```python
from build123d import *

# Parameters (mm, degrees)
BOSS_EXTRUDE1_DEPTH     = 20
BOSS_EXTRUDE4_START     = -30
BOSS_EXTRUDE4_DEPTH     = 42
SKETCH10_W              = 40
SKETCH10_H              = 22
CUT_EXTRUDE3_DEPTH      = 147
SKETCH11_R              = 15
BOSS_EXTRUDE5_DEPTH     = 18
CUT_EXTRUDE4_REACH      = 177
SKETCH12_R              = 10
FILLET1_R               = 3
SKETCH13_R              = 4
CUT_EXTRUDE5_DEPTH      = 86
CUT_EXTRUDE5_DEPTH_BACK = 86
CUT_EXTRUDE7_REACH      = 177
SKETCH16_R              = 6.5


with BuildPart() as part:
    # Sketch1 → Boss-Extrude1 (new body)
    with BuildSketch(Plane(origin=(0, 0, 0), x_dir=(1, 0, 0), z_dir=(0, 1, 0))):
        with BuildLine():
            Line((-80, 30), (80, 30))
            ThreePointArc((80, 30), (83.535533906, 28.535533906), (85, 25))
            Line((85, 25), (85, -25))
            ThreePointArc((85, -25), (83.535533906, -28.535533906), (80, -30))
            Line((80, -30), (-80, -30))
            ThreePointArc((-80, -30), (-83.535533906, -28.535533906), (-85, -25))
            Line((-85, -25), (-85, 25))
            ThreePointArc((-85, 25), (-83.535533906, 28.535533906), (-80, 30))
        make_face()
    extrude(amount=BOSS_EXTRUDE1_DEPTH)

    # Sketch2 → Boss-Extrude4 (add)
    with BuildSketch(Plane.XY.offset(BOSS_EXTRUDE4_START)):
        with BuildLine():
            Line((-17.90827935, 157), (42.09172065, 157))
            Line((42.09172065, 157), (42.09172065, 85))
            Line((42.09172065, 85), (-7.90827935, 85))
            Line((-7.90827935, 85), (-7.90827935, 45))
            Line((-7.90827935, 45), (15, 20))
            Line((15, 20), (37.90827935, 45))
            Line((37.90827935, 45), (42.09172065, 45))
            Line((42.09172065, 45), (42.09172065, 25))
            ThreePointArc((42.09172065, 25), (43.556186744, 21.464466094), (47.09172065, 20))
            Line((47.09172065, 20), (50, 20))
            Line((50, 20), (50, 17))
            Line((50, 17), (-58, 17))
            Line((-58, 17), (-58, 20))
            Line((-58, 20), (-57.90827935, 20))
            ThreePointArc((-57.90827935, 20), (-54.372745445, 21.464466094), (-52.90827935, 25))
            Line((-52.90827935, 25), (-52.90827935, 60))
            ThreePointArc((-52.90827935, 60), (-44.199930596, 92.5), (-20.40827935, 116.291651246))
            ThreePointArc((-20.40827935, 116.291651246), (-18.578152332, 118.121778265), (-17.90827935, 120.621778265))
            Line((-17.90827935, 120.621778265), (-17.90827935, 157))
        make_face()
        with BuildLine():
            Line((-17.90827935, 95.707142143), (-17.90827935, 25))
            ThreePointArc((-17.90827935, 25), (-19.372745445, 21.464466094), (-22.90827935, 20))
            Line((-22.90827935, 20), (-37.90827935, 20))
            ThreePointArc((-37.90827935, 20), (-41.443813256, 21.464466094), (-42.90827935, 25))
            Line((-42.90827935, 25), (-42.90827935, 60))
            ThreePointArc((-42.90827935, 60), (-38.615773866, 81.301408404), (-26.40827935, 99.277856357))
            ThreePointArc((-26.40827935, 99.277856357), (-20.971787677, 100.316914371), (-17.90827935, 95.707142143))
        make_face(mode=Mode.SUBTRACT)
    extrude(amount=BOSS_EXTRUDE4_DEPTH)

    # Sketch10 → Cut-Extrude3 (cut)
    with BuildSketch(Plane(origin=(0, 0, 0), x_dir=(1, 0, 0), z_dir=(0, 1, 0))):
        with Locations((12.09172065, 9)):
            Rectangle(SKETCH10_W, SKETCH10_H)
    extrude(amount=CUT_EXTRUDE3_DEPTH, mode=Mode.SUBTRACT)

    # Sketch11 → Boss-Extrude5 (add)
    with BuildSketch(Plane(origin=(0, 157, 0), x_dir=(1, 0, 0), z_dir=(0, 1, 0))):
        with Locations((12.09172065, 10)):
            Circle(SKETCH11_R)
    extrude(amount=BOSS_EXTRUDE5_DEPTH)

    # Sketch12 → Cut-Extrude4 (cut, up to next)
    with BuildSketch(Plane(origin=(0, 175, 0), x_dir=(1, 0, 0), z_dir=(0, 1, 0)), mode=Mode.PRIVATE) as cut_extrude4_sk1:
        with Locations((12.09172065, 10)):
            Circle(SKETCH12_R)
    cut_extrude4_tool1 = extrude(cut_extrude4_sk1.sketch, amount=-CUT_EXTRUDE4_REACH, mode=Mode.PRIVATE) & part.part
    add(cut_extrude4_tool1.solids().sort_by_distance((12.091721, 175, -10))[0], mode=Mode.SUBTRACT)

    # Fillet1
    fillet1_edges = [part.edges().sort_by_distance(p)[0] for p in [
        (-2.90827935, 157, -10),
        (42.09172065, 85, -9),
        (42.09172065, 157, -9),
        (-17.90827935, 157, -9),
    ]]
    fillet(fillet1_edges, radius=FILLET1_R)

    # Sketch13 → Cut-Extrude5 (cut, two sides)
    with BuildSketch(Plane(origin=(0, 0, 0), x_dir=(0, 0, -1), z_dir=(1, 0, 0))) as cut_extrude5_sk:
        with Locations((10, 140)):
            Circle(SKETCH13_R)
    extrude(amount=CUT_EXTRUDE5_DEPTH, mode=Mode.SUBTRACT)
    extrude(cut_extrude5_sk.sketch, amount=-CUT_EXTRUDE5_DEPTH_BACK, mode=Mode.SUBTRACT)

    # Sketch16 → Cut-Extrude7 (cut, up to next)
    with BuildSketch(Plane(origin=(0, 0, 0), x_dir=(1, 0, 0), z_dir=(0, 1, 0)), mode=Mode.PRIVATE) as cut_extrude7_sk1:
        with Locations((-70, 0)):
            Circle(SKETCH16_R)
    cut_extrude7_tool1 = extrude(cut_extrude7_sk1.sketch, amount=CUT_EXTRUDE7_REACH, mode=Mode.PRIVATE) & part.part
    add(cut_extrude7_tool1.solids().sort_by_distance((-70, 0, 0))[0], mode=Mode.SUBTRACT)
    # Sketch16 → Cut-Extrude7 (cut, up to next)
    with BuildSketch(Plane(origin=(0, 0, 0), x_dir=(1, 0, 0), z_dir=(0, 1, 0)), mode=Mode.PRIVATE) as cut_extrude7_sk2:
        with Locations((70, 0)):
            Circle(SKETCH16_R)
    cut_extrude7_tool2 = extrude(cut_extrude7_sk2.sketch, amount=CUT_EXTRUDE7_REACH, mode=Mode.PRIVATE) & part.part
    add(cut_extrude7_tool2.solids().sort_by_distance((70, 0, 0))[0], mode=Mode.SUBTRACT)


solid = part.part
```
Part model, mm, in its own coordinate system. A direction names the side the tool comes from. Round coordinates to 2 decimals unless told otherwise and drop trailing zeros. Loops run counter-clockwise (first coordinate to the right, second up) from the corner with the lowest first, then second, coordinate; pieces in that order, holes last.
1. Slice it at D-D (z = -10). Count the separate pieces of the cut face and the enclosed holes in it, and give its area (3 significant figures).
Solutions:
separate pieces: 5
enclosed holes: 1
area: 6,220 mm2
2. Slice it at C-C (y = 48). Give the cut face in (x, z).
Solutions:
outline: (-52.91, -30) - (-42.91, -30) - (-42.91, 12) - (-52.91, 12) - close; (-17.91, -30) - (-7.91, -30) - (-7.91, 12) - (-17.91, 12) - close
3. Drill centre lines: line 1 along X through (y, z) = (36, -15); line 2 along X through (y, z) = (7, 0); line 3 along X through (y, z) = (160.25, -10). Where is each one in solid material? Low to high.
Solutions:
line 1: x = -52.91 to -42.91, -17.91 to -7.91, 32.09 to 42.09
line 2: x = -85 to -76.5, -63.5 to -7.91, 32.09 to 63.5, 76.5 to 85
line 3: x = -2.91 to 2.09, 22.09 to 27.09
4. Flat gauge pins, fed straight in: pin 1 (1 mm diameter, centred on y = 116.5, z = -16.5, fed in from -X); pin 2 (8 mm diameter, centred on y = 91.5, z = 1, fed in from +X); pin 3 (18 mm diameter, centred on x = 12.09, z = -10, fed in from -Y); pin 4 (1.3 mm diameter, centred on x = 40.5, z = -6.5, fed in from +Y). Where does each tip first touch, or does it go through?
Solutions:
pin 1: stops at x = -20.91
pin 2: stops at x = 42.09
pin 3: passes through
pin 4: stops at y = 156.9
5. 3-axis set-ups, long thin cutter, end or side, ignore diameter. For faces 4 (the face through (16, 85, -23)), 5 (the face through (12, 17, -20)), 6 (the face through (-52.908, 42, -9)): which of +Z, -Z, +X, -X, +Y, -Y reach the whole face in a straight line?
Solutions:
face 4: +Z, -Z, +X
face 5: -Y
face 6: +Z, -Z, -X, +Y
6. Two-plate mould, pull along X, no slides. Class faces 1 (the face through (84, 10, 28)), 2 (the face through (-38.734, 81.019, -9.294)), 3 (the face through (-12.838, 143.966, -9.479)): pulls with the +X half, pulls with the -X half, needs draft (parallel to the pull), parting line crosses it, or undercut.
Solutions:
face 1: pulls with the +X half
face 2: undercut
face 3: needs draft
7. Slice it at B-B (x = 70). Give the cut face in (y, z).
Solutions:
outline: (0, -30) - (20, -30) - (20, -6.5) - (0, -6.5) - close; (0, 6.5) - (20, 6.5) - (20, 30) - (0, 30) - close
8. Slice it at A-A (y = 140). Give the cut face in (x, z), and give its area (3 significant figures).
Solutions:
outline: (-17.91, -30) - (42.09, -30) - (42.09, -14) - (32.09, -14) - (32.09, -20) - (-7.91, -20) - (-7.91, -14) - (-17.91, -14) - close; (-17.91, -6) - (-7.91, -6) - (-7.91, 2) - (32.09, 2) - (32.09, -6) - (42.09, -6) - (42.09, 12) - (-17.91, 12) - close
area: 1,480 mm2
